For this review, take the finished solid that the model builds, in its own axes (mm). A direction names the side the tool comes from. Round coordinates to 2 decimals unless told otherwise and drop trailing zeros. Write each loop counter-clockwise with the first axis right and the second up, starting at its lowest first coordinate (ties: lowest second). Pieces come first, ordered by that corner, then holes. Notation, with made-up numbers: (-6.75, 33) -> (52.25, 33) arc R19 cw to (52.25, 39) -> close; hole circle Ø10 at (45.25, -37.75). An arc over 180 degrees is marked (long way). Answer in a Markdown table with one row per item.
from build123d import *

# Parameters (mm, degrees)
F0_R      = 33.5
F0_R_2    = 30
F1_DEPTH  = 40
F2_DEPTH  = 5
F4_R      = 22.5
F5_DEPTH  = 15
F6_R      = 9.648843
F7_DEPTH  = 25
F9_R      = 39.178288
F10_DEPTH = 25


with BuildPart() as f1:
    # F0 (on Top) → F1 (new body)
    with BuildSketch(Plane.XY):
        Circle(F0_R)
        Circle(F0_R_2, mode=Mode.SUBTRACT)
        Circle(F0_R_2)
    extrude(amount=F1_DEPTH)

    # F0 (on Top) → F2 (cut)
    with BuildSketch(Plane.XY):
        Circle(F0_R_2)
    extrude(amount=F2_DEPTH, mode=Mode.SUBTRACT)

    # F4 (on face) → F5 (cut)
    with BuildSketch(Plane.XY):
        Circle(F4_R)
    extrude(amount=F5_DEPTH, mode=Mode.SUBTRACT)

    # F6 (on face) → F7 (join)
    with BuildSketch(Plane.XY.offset(40)):
        Circle(F6_R)
    extrude(amount=F7_DEPTH)

    # F9 (on offset) → F10 (join)
    with BuildSketch(Plane.XY.offset(10)):
        Circle(F9_R)
    extrude(amount=F10_DEPTH)


solid = f1.part
1) For line 1 (X direction, y = 0, z = 6.35); line 2 (Y direction, x = 0, z = 3); line 3 (Z direction, x = -1, y = -12), list the stretches that pass through material, from the lowest coordinate up. Write a range as [from, to].
Solved:
| item | result |
|---|---|
| line 1 | [-33.5, -22.5], [22.5, 33.5] |
| line 2 | [-33.5, -30], [30, 33.5] |
| line 3 | [10, 40] |
2) Clearance check with flat-ended pins moving along their axes: pin 1 Ø6 at (x, y) = (22, -13.5) entering from -Z; pin 2 Ø8 at (x, z) = (-25, 41) entering from +Y; pin 3 Ø6 at (x, z) = (-8, 14) entering from +Y. State where each tip first meets the part, or that it passes through.
Solved:
| item | result |
|---|---|
| pin 1 | z = 5 |
| pin 2 | y = 26 |
| pin 3 | y = 38.86 |
3) Consider section A-A on x = 0. State the section outline as (y, z) points.
Solved:
| item | result |
|---|---|
| outline | (-39.18, 10) -> (-33.5, 10) -> (-33.5, 0) -> (-30, 0) -> (-30, 5) -> (-22.5, 5) -> (-22.5, 10) -> (22.5, 10) -> (22.5, 5) -> (30, 5) -> (30, 0) -> (33.5, 0) -> (33.5, 10) -> (39.18, 10) -> (39.18, 35) -> (33.5, 35) -> (33.5, 40) -> (9.65, 40) -> (9.65, 65) -> (-9.65, 65) -> (-9.65, 40) -> (-33.5, 40) -> (-33.5, 35) -> (-39.18, 35) -> close |
4) Consider section C-C on z = 49.5. State the section outline as (x, y) points.
Solved:
| item | result |
|---|---|
| outline | circle Ø19.3 at (0, 0) |
5) Consider section D-D on y = 25. State the section outline as (x, z) points, then the cut area to 3 significant figures.
Solved:
| item | result |
|---|---|
| outline | (-30.17, 10) -> (-22.3, 10) -> (-22.3, 0) -> (-16.58, 0) -> (-16.58, 5) -> (16.58, 5) -> (16.58, 0) -> (22.3, 0) -> (22.3, 10) -> (30.17, 10) -> (30.17, 35) -> (22.3, 35) -> (22.3, 40) -> (-22.3, 40) -> (-22.3, 35) -> (-30.17, 35) -> close |
| area | 2,010 mm² |
6) Mouldability with a two-part tool opening along Y and no side actions: class faces 1 (the cylindrical face through (10.382, -19.961, 7.465)), 2 (the flat face through (7, -7, 40)), 3 (the cylindrical face through (-7.262, -32.703, 37.465)) as pulls with the +Y half, pulls with the -Y half, needs draft (parallel to the pull), parting line crosses it, or undercut.
Solved:
| item | result |
|---|---|
| face 1 | undercut |
| face 2 | needs draft |
| face 3 | parting line crosses it |
7) For faces 4 (the flat face through (29, 18, 35)), 5 (the cylindrical face through (37.37, 11.77, 22.32)), 6 (the cylindrical face through (-29.97, 1.32, 2.46)), list the 3-axis set-ups (+Z, -Z, +X, -X, +Y, -Y) from which the entire face can be reached by the end or side of a thin tool; tool diameter is ignored.
Solved:
| item | result |
|---|---|
| face 4 | +Z |
| face 5 | +Z, -Z |
| face 6 | -Z |
